Read the model definition and answer for the solid it produces. Units are mm, in the model's axes. Coordinates: 2 decimals unless noted, no trailing zeros. Write each loop counter-clockwise with the first axis right and the second up, starting at its lowest first coordinate (ties: lowest second). Pieces come first, ordered by that corner, then holes. Notation, with made-up numbers: (22, 82) -> (46, 82) arc R18 ccw to (46, 112) -> close; hole circle Ø5 at (22.5, 33.25). An arc over 180 degrees is marked (long way). Use CSV: the item, a comma, the result in double quotes.
Autodesk Inventor part; units mm, degrees
ref_plane "YZ Plane" through (0, 0, 0) normal (1, 0, 0) x (0, 1, 0)
ref_plane "XZ Plane" through (0, 0, 0) normal (0, 1, 0) x (-1, 0, 0)
ref_plane "XY Plane" through (0, 0, 0) normal (0, 0, 1) x (1, 0, 0)
sketch "Szkic1" plane through (0, 0, 0) normal (0, 0, 1) x (1, 0, 0)
  line L0 (-25.3316, -15.5729) -> (26.0684, -15.5729)
  line L1 (26.0684, -15.5729) -> (26.0684, 35.4271)
  line L2 (26.0684, 35.4271) -> (26.0684, 35.4271)
  line L3 (26.0684, 35.4271) -> (26.0684, 55.4271)
  line L4 (26.0684, 55.4271) -> (-5.3316, 55.4271)
  line L5 (-5.3316, 55.4271) -> (-5.3316, 86.8271)
  line L6 (-5.3316, 86.8271) -> (-25.3316, 86.8271)
  line L7 (-25.3316, -15.5729) -> (-25.3316, 86.8271)
  line L8 (-15.6316, 16.9271) -> (16.3684, 16.9271)
  line L9 (16.3684, 16.9271) -> (16.3684, -15.0729)
  line L10 (16.3684, -15.0729) -> (-15.6316, -15.0729)
  line L11 (-15.6316, -15.0729) -> (-15.6316, 16.9271)
  circle A0 centre (0.3684, 0.9271) radius 11
  circle A1 centre (0.3684, 0.9271) radius 16
  point P0 (0, 0)
  point P1 (-10.9453, 12.2408)
  point P2 (11.6821, 12.2408)
  point P3 (11.6821, -10.3866)
  point P4 (-10.9453, -10.3866)
  point P5 (16.0684, 45.4271)
  point P6 (-15.3316, 76.8271)
  point P7 (-15.3316, 45.4271)
  dimension "d0" = 20
  dimension "d1" = 20
  dimension "d2" = 51.4
  dimension "d3" = 51.4
  dimension "d4" = 34.5
  dimension "d5" = 25.7
  dimension "d6" = 51.4
  dimension "d7" = 51
  dimension "d8" = 32
  dimension "d9" = 32
  dimension "d10" = 16
  dimension "d11" = 16
  dimension "d12" = 22
  dimension "d13" = 32
  dimension "d23" = 10
  dimension "d24" = 10
  dimension "d25" = 10
  dimension "d26" = 10
  dimension "d27" = 10
  dimension "d28" = 10
extrude "Wyciągnięcie proste1" add sketch "Szkic1" along normal blind 4 contours L7 L6 L5 L4 L3 L1 L0 | L8 A1 L11 | L8 L9 A1 | A1 | A1 L10 L11 | L9 L10 A1
hole "Otwór1" at (0.3684, 0.9271, 0) at (-10.9453, 12.2408, 0) at (11.6821, 12.2408, 0) at (11.6821, -10.3866, 0) at (-10.9453, -10.3866, 0) direction (0, 0, 1) diameter 4 end through all
hole "Otwór2" at (16.0684, 45.4271, 0) at (-15.3316, 76.8271, 0) at (-15.3316, 45.4271, 0) direction (0, 0, 1) diameter 4 end through all
chamfer "Faza1" distance 51 distance2 9.7 1 edges at (-25.3316, -15.5729, 2) measured on face at (-25.3316, 18.5605, 1.3333)
chamfer "Faza2" distance 51 distance2 9.7 1 edges at (26.0684, -15.5729, 2) measured on face at (26.0684, 31.7605, 1.3333)
fillet "Zaokrąglenie2" radius 6 4 edges at (-5.3316, 55.4271, 2) (26.0684, 55.4271, 2) (-5.3316, 86.8271, 2) (-25.3316, 86.8271, 2)
fillet "Zaokrąglenie3" radius 10 2 edges at (-25.3316, 35.4271, 2) (26.0684, 35.4271, 2)
sketch "Szkic2" plane through (0, 0, 4) normal (0, 0, 1) x (1, 0, 0)
  arc A0 (25.8923, 34.5012) -> (26.0684, 36.3697) centre (16.0684, 36.3697) ccw
  line L0 (26.0684, 36.3697) -> (26.0684, 49.4271)
  arc A1 (26.0684, 49.4271) -> (20.0684, 55.4271) centre (20.0684, 49.4271) ccw
  line L1 (20.0684, 55.4271) -> (0.6684, 55.4271)
  arc A2 (-5.3316, 61.4271) -> (0.6684, 55.4271) centre (0.6684, 61.4271) ccw
  line L2 (-5.3316, 61.4271) -> (-5.3316, 80.8271)
  arc A3 (-5.3316, 80.8271) -> (-11.3316, 86.8271) centre (-11.3316, 80.8271) ccw
  line L3 (-11.3316, 86.8271) -> (-19.3316, 86.8271)
  arc A4 (-19.3316, 86.8271) -> (-25.3316, 80.8271) centre (-19.3316, 80.8271) ccw
  line L4 (-25.3316, 80.8271) -> (-25.3316, 36.3697)
  arc A5 (-25.3316, 36.3697) -> (-25.1555, 34.5012) centre (-15.3316, 36.3697) ccw
  line L5 (-15.6316, -15.5729) -> (-25.1555, 34.5012)
  line L6 (-15.6316, -15.5729) -> (16.3684, -15.5729)
  line L7 (25.8923, 34.5012) -> (16.3684, -15.5729)
  circle A6 centre (-15.3316, 76.8271) radius 2
  circle A7 centre (16.0684, 45.4271) radius 2
  circle A8 centre (-15.3316, 45.4271) radius 2
  circle A9 centre (11.6821, -10.3866) radius 2
  circle A10 centre (-10.9453, 12.2408) radius 2
  circle A11 centre (11.6821, 12.2408) radius 2
  circle A12 centre (-10.9453, -10.3866) radius 2
  circle A13 centre (0.3684, 0.9271) radius 11
  line L8 (-17.3434, -6.5729) -> (-48.8316, -6.5729)
  line L9 (-48.8316, -6.5729) -> (-48.8316, 8.4271)
  line L10 (-48.8316, 8.4271) -> (-20.1963, 8.4271)
  point P0 (0, 0)
  point P1 (-42.8316, 0.9271)
  dimension "d45" = 15
  dimension "d46" = 9
  dimension "d47" = 23.5
  dimension "d50" = 7.5
  dimension "d51" = 6
extrude "Wyciągnięcie proste2" add sketch "Szkic2" against normal blind 4 contours L8 L9 L10 L5
hole "Otwór3" at (-42.8316, 0.9271, 4) direction (0, 0, -1) diameter 3 end through all
fillet "Zaokrąglenie4" radius 8 4 edges at (-17.3434, -6.5729, 2) (-20.1963, 8.4271, 2) (-48.8316, -6.5729, 2) (-48.8316, 8.4271, 2)
fillet "Zaokrąglenie5" radius 2 2 edges at (-15.6316, -15.5729, 2) (16.3684, -15.5729, 2)
equation "\"d1\" = d0"
equation "\"d2\" = d6"
equation "\"d3\" = d6"
equation "\"d6\" = 2 * d5"
properties part number "LC_ALU_4mm_Heatbed_Frame_Linear_Bearing_Mounting_Bracket_Z_endstop"
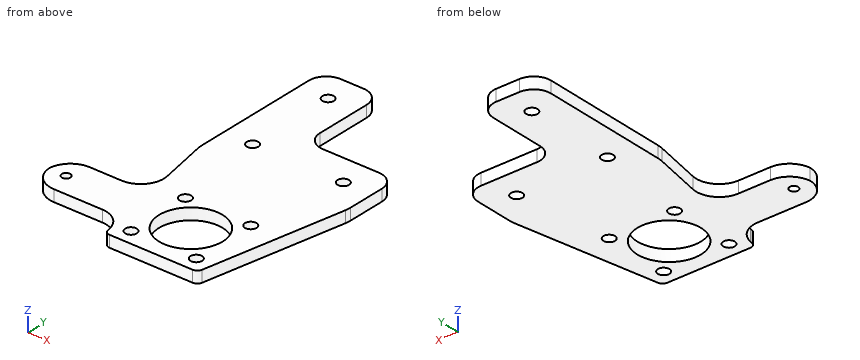
1. A cutting plane is placed at B-B (z = 0.8). Give the number of separate pieces and of enclosed holes in the cut face, and give its area (3 significant figures).
Solutions:
separate pieces,"1"
enclosed holes,"9"
area,"3,740 mm^2"
2. Find the intervals of material crossed by line 1 along Y through (x, z) = (-30, 3.6); line 2 along X through (y, z) = (77.5, 3.2) (3 decimals); line 3 along Y through (x, z) = (-11.5, 3.6), in increasing order.
Solutions:
line 1,"y = -6.57 to 8.43"
line 2,"x = -25.332 to -17.215, -13.448 to -5.332"
line 3,"y = -15.57 to -12.31, -8.47 to 10.32, 14.16 to 86.83"
3. A cutting plane is placed at D-D (y = 45.5). Give the vertices of the cut face in (x, z).
Solutions:
outline,"(-25.33, 0) -> (-17.33, 0) -> (-17.33, 4) -> (-25.33, 4) -> close; (-13.33, 0) -> (14.07, 0) -> (14.07, 4) -> (-13.33, 4) -> close; (18.07, 0) -> (26.07, 0) -> (26.07, 4) -> (18.07, 4) -> close"
4. Each of these flat-tipped pins is pushed along its axis until it touches: pin 1 Ø1.2 at (x, z) = (-33.5, 3) entering from +Y; pin 2 Ø2 at (x, z) = (14, 1) entering from +Y; pin 3 Ø3.5 at (x, y) = (11.68, 12.24) entering from +Z; pin 4 Ø2 at (y, z) = (71.5, 1) entering from +X. Where does it stop, or does it pass through?
Solutions:
pin 1,"stops at y = 8.43"
pin 2,"stops at y = 55.43"
pin 3,"passes through"
pin 4,"stops at x = -5.33"
5. A cutting plane is placed at C-C (y = 4). Give the vertices of the cut face in (x, z), and give its area (3 significant figures).
Solutions:
outline,"(-48.05, 0) -> (-10.19, 0) -> (-10.19, 4) -> (-48.05, 4) -> close; (10.93, 0) -> (20.09, 0) -> (20.09, 4) -> (10.93, 4) -> close"
area,"188 mm^2"
6. A cutting plane is placed at A-A (x = 6). Give the vertices of the cut face in (y, z).
Solutions:
outline,"(-15.57, 0) -> (-8.52, 0) -> (-8.52, 4) -> (-15.57, 4) -> close; (10.38, 0) -> (55.43, 0) -> (55.43, 4) -> (10.38, 4) -> close"
